Read the model definition and answer for the solid it produces. Units are mm, in the model's axes. A direction names the side the tool comes from. Give positions to 0.01 mm unless a question says otherwise; leave off trailing zeros. Order: outer loops, then holes, each group sorted by start corner. A loop starts at its lowest first (then second) coordinate and runs counter-clockwise, first axis right, second up. Notation, with made-up numbers: (17, 57) - (58, 57) arc R7 cw to (58, 66) - close; hole circle Ø1 at (22.25, 14). An arc over 180 degrees is marked (long way). Use a Markdown table: item, result. Add a question column.
1. Which of the six approach directions +Z, -Z, +X, -X, +Y, -Y give full straight-line access (tool end or side, diameter ignored) to faces 1 (the flat face through (-2, -15, 3)), 2 (the flat face through (10, -166.5, 3)), 3 (the flat face through (70, -27, 3)), 4 (the flat face through (4, -171.5, 3)), 5 (the flat face through (72, -185, 3))?
2. Consider L1, parallel to X at y = -27, z = 1.85; L2, parallel to Y at x = 11.4, z = 4.3; L3, parallel to Y at x = 7, z = 5.3. Determine where each line is inside the solid, lowest interval first.
3. Flat-ended cylindrical pins translate along their axes: P1, Ø2.5, axis at x = 73, z = 4, coming from the -Y side; P2, Ø2, axis at y = -173, z = 4, coming from the -X side; P3, Ø1.5, axis at x = 72.5, z = 2, coming from the +Y side. Find the tip coordinate at first contact, or state that the pin passes through.
4. A cutting plane is placed at B-B on z = 1.9. State how many separate pieces and enclosed holes the cut face has, and give its area (3 significant figures).
5. A cutting plane is placed at A-A on y = -119. Determine the outline of the cut face in (x, z), and give its area (3 significant figures).
6. For a pull along X with two mould halves and no side action, classify faces 6 (the flat face through (0, -192, 3)), 7 (the flat face through (60, -173.5, 3)), 8 (the flat face through (75, -40, 3)) as released by +X, released by -X, zero draft, split by the parting line, or undercut.
```python
from build123d import *

# Parameters (mm, degrees)
MODEL_R                  = 1.25
MODEL_R_2                = 6
RESSALTO_EXTRUS_O1_DEPTH = 6


with BuildPart() as part:
    # Model → Ressalto-extrusão1 (new body)
    with BuildSketch(Plane.XY):
        Polygon((70, -31.5), (62, -31.5), (62, -33.5), (57, -33.5), (57, -26.5), (62, -26.5), (62, -28.5), (70, -28.5), (70, -25), (75, -25), (75, -15), (70, -15), (70, 0), (0, 0), (0, -15), (-5, -15), (-5, -25), (0, -25), (0, -28.5), (8, -28.5), (8, -26.5), (13, -26.5), (13, -33.5), (8, -33.5), (8, -31.5), (0, -31.5), (0, -35), (-5, -35), (-5, -45), (0, -45), (0, -155), (-5, -155), (-5, -165), (0, -165), (0, -168.5), (8, -168.5), (8, -166.5), (13, -166.5), (13, -173.5), (8, -173.5), (8, -171.5), (0, -171.5), (0, -175), (-5, -175), (-5, -185), (0, -185), (0, -200), (70, -200), (70, -185), (75, -185), (75, -175), (70, -175), (70, -171.5), (62, -171.5), (62, -173.5), (57, -173.5), (57, -166.5), (62, -166.5), (62, -168.5), (70, -168.5), (70, -165), (75, -165), (75, -155), (70, -155), (70, -45), (75, -45), (75, -35), (70, -35), align=None)
        with Locations((32.177, -78.842)):
            Circle(MODEL_R, mode=Mode.SUBTRACT)
        with Locations((35.353, -69)):
            Circle(MODEL_R, mode=Mode.SUBTRACT)
        with Locations((32.177, -59.158)):
            Circle(MODEL_R, mode=Mode.SUBTRACT)
        with Locations((18.403, -52.05)):
            Circle(MODEL_R, mode=Mode.SUBTRACT)
        with Locations((4.629, -59.158)):
            Circle(MODEL_R, mode=Mode.SUBTRACT)
        with Locations((4.629, -78.842)):
            Circle(MODEL_R, mode=Mode.SUBTRACT)
        with Locations((18.403, -85.95)):
            Circle(MODEL_R, mode=Mode.SUBTRACT)
        with Locations((11.4, -69)):
            Circle(MODEL_R_2, mode=Mode.SUBTRACT)
    extrude(amount=RESSALTO_EXTRUS_O1_DEPTH)


solid = part.part
```
Output values:
| question | item | result |
|---|---|---|
| 1 | face 1 | +Z, -Z, -X, +Y |
| 1 | face 2 | +Z, -Z |
| 1 | face 3 | +Z, -Z, +X |
| 1 | face 4 | +Z, -Z, -X |
| 1 | face 5 | +Z, -Z, +X, -Y |
| 2 | L1 | 0 to 8, 13 to 57, 62 to 70 |
| 2 | L2 | -200 to -173.5, -166.5 to -75, -63 to -33.5, -26.5 to 0 |
| 2 | L3 | -200 to -171.5, -168.5 to -73.08, -64.92 to -31.5, -28.5 to 0 |
| 3 | P1 | y = -185 |
| 3 | P2 | x = 0 |
| 3 | P3 | y = -15 |
| 4 | separate pieces | 1 |
| 4 | enclosed holes | 8 |
| 4 | area | 14,000 mm² |
| 5 | outline | (0, 0) - (70, 0) - (70, 6) - (0, 6) - close |
| 5 | area | 420 mm² |
| 6 | face 6 | released by -X |
| 6 | face 7 | undercut |
| 6 | face 8 | released by +X |
